```python
from build123d import *

# Parameters (mm, degrees)
SKETCH1_R           = 6
BOSS_EXTRUDE1_DEPTH = 100
SKETCH2_R           = 3
CUT_EXTRUDE1_DEPTH  = 30
SKETCH3_R           = 3
CUT_EXTRUDE2_DEPTH  = 60


with BuildPart() as part:
    # Sketch1 → Boss-Extrude1 (new body)
    with BuildSketch(Plane(origin=(0, 0, 0), x_dir=(0, 0, -1), z_dir=(1, 0, 0))):
        Circle(SKETCH1_R)
    extrude(amount=BOSS_EXTRUDE1_DEPTH)

    # Sketch2 → Cut-Extrude1 (cut)
    with BuildSketch(Plane(origin=(100, 0, 0), x_dir=(0, 0, -1), z_dir=(1, 0, 0))):
        Circle(SKETCH2_R)
    extrude(amount=-CUT_EXTRUDE1_DEPTH, mode=Mode.SUBTRACT)

    # Sketch3 → Cut-Extrude2 (cut)
    with BuildSketch(Plane.ZY):
        Circle(SKETCH3_R)
    extrude(amount=-CUT_EXTRUDE2_DEPTH, mode=Mode.SUBTRACT)


solid = part.part
```
Geometry: final body of the model. Coordinates: model frame, mm. A direction names the side the tool comes from. Round coordinates to 2 decimals unless told otherwise and drop trailing zeros. Write each loop counter-clockwise with the first axis right and the second up, starting at its lowest first coordinate (ties: lowest second). Pieces come first, ordered by that corner, then holes.
Item 1: Section query A-A (y = 0). Return loops of the section in (x, z), plus the area to 3 significant figures.
Item 2: Section query D-D (x = 63.5). Return loops of the section in (y, z).
Item 3: Mould query, pull axis Z, two halves, no side actions, for faces 4 (the face through (0, -1, 3)), 5 (the face through (49, 0, 6)), 6 (the face through (30, 0, -3)). Classes: +Z half, -Z half, draft (parallel to the pull), parting line (faces both ways), or undercut.
Item 4: Material intervals for L1, parallel to Y at x = 77, z = 0; L2, parallel to X at y = 0.5, z = 2.5; L3, parallel to Z at x = 51, y = 1, sorted ascending.
Item 5: Section query B-B (x = 14). Return loops of the section in (y, z).
Item 6: Pin query (flat end, axial travel): P1, Ø1.8, axis at y = -0.5, z = 0.5, coming from the -X side; P2, Ø5.5, axis at y = 0, z = 0, coming from the +X side; P3, Ø1.5, axis at x = 88, y = -3.5, coming from the +Z side. Return the tip coordinate at first contact, or that it passes through.
Item 7: Section query C-C (z = -0.25). Return loops of the section in (x, y).
Item 8: Set-up query: faces 1 (the face through (60, 0, 0)), 2 (the face through (85, 0, 3)), 3 (the face through (100, -1, 3)). Return all of +Z, -Z, +X, -X, +Y, -Y with unobstructed straight access to the full face (end or side cutting, diameter ignored); none if empty.
Completed:
1. outline: (0, -6) - (100, -6) - (100, -3) - (70, -3) - (70, 3) - (100, 3) - (100, 6) - (0, 6) - (0, 3) - (60, 3) - (60, -3) - (0, -3) - close
1. area: 660 mm2
2. outline: circle Ø12 at (0, 0)
3. face 4: draft
3. face 5: parting line
3. face 6: undercut
4. L1: y = -6 to -3, 3 to 6
4. L2: x = 60 to 70
4. L3: z = -5.92 to -2.83, 2.83 to 5.92
5. outline: circle Ø12 at (0, 0); hole circle Ø6 at (0, 0)
6. P1: stops at x = 60
6. P2: stops at x = 70
6. P3: stops at z = 5.33
7. outline: (0, -5.99) - (100, -5.99) - (100, -2.99) - (70, -2.99) - (70, 2.99) - (100, 2.99) - (100, 5.99) - (0, 5.99) - (0, 2.99) - (60, 2.99) - (60, -2.99) - (0, -2.99) - close
8. face 1: -X
8. face 2: +X
8. face 3: +Z, -Z, +X, +Y, -Y
